from build123d import *

# Parameters (mm, degrees)
F0_R      = 9.525
F1_DEPTH  = 15.8115
F2_R      = 11.1125
F3_DEPTH  = 7.112
F4_R      = 11.1125
F5_DEPTH  = 7.112
F6_T      = 3.175
F7_R      = 3.175
F8_DEPTH  = 3.175
F10_R     = 11.1125
F11_DEPTH = 1.5875
F12_W     = 13.096875
F12_H     = 13.096875
F13_DEPTH = 15.8115
F14_R     = 4.7625
F15_R     = 8.334375


# Not quite as in the source:
# - a shell that OpenCascade refuses in one call is made with other operations: the cavity is built on its own and cut out


with BuildPart() as f1:
    # F0 (on Top) → F1 (new body)
    with BuildSketch(Plane.XY):
        with BuildLine():
            Line((-14.2875, 369.1638474552), (-14.2875, 0))
            ThreePointArc((-14.2875, 0), (-13.1999288208, -5.4675895399), (-10.1027881362, -10.1027881362))
            Line((-10.1027881362, -10.1027881362), (23.8125, -44.0180762724))
            Line((23.8125, -44.0180762724), (74.6125, -44.0180762724))
            Line((74.6125, -44.0180762724), (74.6125, 413.1819237276))
            Line((74.6125, 413.1819237276), (23.8125, 413.1819237276))
            Line((23.8125, 413.1819237276), (-10.1027881362, 379.2666355914))
            ThreePointArc((-10.1027881362, 379.2666355914), (-13.1999288208, 374.6314369951), (-14.2875, 369.1638474552))
        make_face()
        Circle(F0_R, mode=Mode.SUBTRACT)
        with Locations((0, 369.1638474552)):
            Circle(F0_R, mode=Mode.SUBTRACT)
    extrude(amount=F1_DEPTH)

    # F2 (on face) → F3 (cut)
    with BuildSketch(Plane.XY.offset(15.8115)):
        with Locations((0, 369.1638474552)):
            Circle(F2_R)
        Circle(F2_R)
    extrude(amount=-F3_DEPTH, mode=Mode.SUBTRACT)

    # F4 (on face) → F5 (cut)
    with BuildSketch(Plane(origin=(0, 0, 0), x_dir=(1, 0, 0), z_dir=(0, 0, -1))):
        Circle(F4_R)
        with Locations((0, -369.1638474552)):
            Circle(F4_R)
    extrude(amount=-F5_DEPTH, mode=Mode.SUBTRACT)

    # F6: shell of thickness 3.175, made by hand


with BuildPart() as f6_core1:
    # F6_t2: copy of F1
    add(f1.part)

    # the walls: a layer under each face that stays
    f6_faces = [f6_core1.faces().sort_by_distance(p)[0] for p in [
        (-13.1999288208, 374.6314369951, 7.90575),
        (6.8548559319, 396.2242796595, 7.90575),
        (-14.2875, 184.5819237276, 7.90575),
        (30.1625, 184.5819237276, 15.8115),
        (49.2125, 413.1819237276, 7.90575),
        (-13.1999288208, -5.4675895399, 7.90575),
        (74.6125, 184.5819237276, 7.90575),
        (6.8548559319, -27.0604322043, 7.90575),
        (49.2125, -44.0180762724, 7.90575),
        (-11.1125, 0, 3.556),
        (-11.1125, 369.1638474552, 3.556),
        (-11.1125, 0, 12.2555),
        (-11.1125, 369.1638474552, 12.2555),
        (-7.4083333333, 7.4083333333, 7.112),
        (-7.4083333333, 376.5721807885, 7.112),
        (-7.4083333333, -7.4083333333, 8.6995),
        (-7.4083333333, 361.7555141219, 8.6995),
        (-9.525, 0, 7.90575),
        (-9.525, 369.1638474552, 7.90575),
    ]]
    thicken(f6_faces, amount=-F6_T, mode=Mode.SUBTRACT)

    # F6_s3 → F6_t4 (revolve, cut)
    with BuildSketch(Plane.XZ):
        Polygon((11.08075, 7.08025), (14.2875, 7.112), (14.2875, 10.287), (11.1125, 10.287), align=None)
    revolve(axis=Axis((0, 0, 7.112), (0, 0, -1)), mode=Mode.SUBTRACT)

    # F6_s5 → F6_t6 (revolve, cut)
    with BuildSketch(Plane.XZ.offset(-369.1638474552)):
        Polygon((11.08075, 7.08025), (14.2875, 7.112), (14.2875, 10.287), (11.1125, 10.287), align=None)
    revolve(axis=Axis((0, 369.1638474552, 7.112), (0, 0, -1)), mode=Mode.SUBTRACT)

    # F6_s7 → F6_t8 (revolve, cut)
    with BuildSketch(Plane.XZ):
        Polygon((11.08075, 8.73125), (14.2875, 8.6995), (14.2875, 5.5245), (11.1125, 5.5245), align=None)
    revolve(axis=Axis((0, 0, 8.6995), (0, 0, 1)), mode=Mode.SUBTRACT)

    # F6_s9 → F6_t10 (revolve, cut)
    with BuildSketch(Plane.XZ.offset(-369.1638474552)):
        Polygon((11.08075, 8.73125), (14.2875, 8.6995), (14.2875, 5.5245), (11.1125, 5.5245), align=None)
    revolve(axis=Axis((0, 369.1638474552, 8.6995), (0, 0, 1)), mode=Mode.SUBTRACT)


with BuildPart() as f1_1:
    add(f1.part)

    # what is left inside the walls is the cavity
    f6_cavity = [f6_core1.part.solids().sort_by_distance(p)[0] for p in [
        (30.1625, 109.440257, 12.60475),
    ]]
    add(f6_cavity, mode=Mode.SUBTRACT)

    # F7
    f7_edges = [f1_1.edges().sort_by_distance(p)[0] for p in [
        (-1.507724, 383.371572, 6.31825),
        (-11.1125, 360.183591, 6.31825),
        (-11.1125, 8.980256, 6.31825),
        (-1.507724, -14.207724, 6.31825),
    ]]
    fillet(f7_edges, radius=F7_R)

    # F8 (cut, through all): a face of the model
    f8_faces = [f1_1.faces().sort_by_distance(p)[0] for p in [
        (32.2546535053, 184.5819237276, 12.6365),
    ]]
    extrude(f8_faces, amount=-F8_DEPTH, mode=Mode.SUBTRACT)

    # F10 (on offset) → F11 (join, symmetric)
    with BuildSketch(Plane.XY.offset(7.90575)):
        with BuildLine():
            Line((74.6125, -44.0180762724), (74.6125, 413.1819237276))
            Line((74.6125, 413.1819237276), (23.8125, 413.1819237276))
            Line((23.8125, 413.1819237276), (-10.1027881362, 379.2666355914))
            ThreePointArc((-10.1027881362, 379.2666355914), (-13.1999288208, 374.6314369951), (-14.2875, 369.1638474552))
            Line((-14.2875, 369.1638474552), (-14.2875, 0))
            ThreePointArc((-14.2875, 0), (-13.1999288208, -5.4675895399), (-10.1027881362, -10.1027881362))
            Line((-10.1027881362, -10.1027881362), (23.8125, -44.0180762724))
            Line((23.8125, -44.0180762724), (74.6125, -44.0180762724))
        make_face()
        Circle(F10_R, mode=Mode.SUBTRACT)
        with Locations((0, 369.1638474552)):
            Circle(F10_R, mode=Mode.SUBTRACT)
    extrude(amount=F11_DEPTH, both=True)

    # F12 (on face) → F13 (join, through all)
    with BuildSketch(Plane(origin=(0, 0, 0), x_dir=(1, 0, 0), z_dir=(0, 0, -1))):
        with Locations((68.0640625, -406.6334862276)):
            Rectangle(F12_W, F12_H)
        with Locations((68.0640625, 37.4696387724)):
            Rectangle(F12_W, F12_H)
    extrude(amount=-F13_DEPTH)

    # F14
    f14_edges = [f1_1.edges().sort_by_distance(p)[0] for p in [
        (61.515625, 400.085049, 12.652375),
        (61.515625, 400.085049, 3.159125),
        (61.515625, -30.921201, 12.652375),
        (61.515625, -30.921201, 3.159125),
    ]]
    fillet(f14_edges, radius=F14_R)

    # F15
    f15_edges = [f1_1.edges().sort_by_distance(p)[0] for p in [
        (74.6125, -44.018076, 7.90575),
        (74.6125, 413.181924, 7.90575),
    ]]
    fillet(f15_edges, radius=F15_R)


solid = f1_1.part
The model under review builds one solid part; all positions refer to its coordinate system, in mm. A direction names the side the tool comes from. Round coordinates to 2 decimals unless told otherwise and drop trailing zeros. Write each loop counter-clockwise with the first axis right and the second up, starting at its lowest first coordinate (ties: lowest second). Pieces come first, ordered by that corner, then holes. Notation, with made-up numbers: (64, -29.5) - (115, -29.5) arc R7 cw to (115, -25.5) - close; hole circle Ø3 at (42, 61.25). An arc over 180 degrees is marked (long way). One line per item, written item: value. Start each with the question number.
1. Machinability: for faces 1 (the face through (74.612, 181, 8)), 2 (the face through (13.323, 5.161, 3.203)), 3 (the face through (-5, 8.3, 8.7)), which of the approach directions +Z, -Z, +X, -X, +Y, -Y give a long, thin tool a straight path to every point of the face, cutting with its end or side? Answer none if there is none.
2. To check wall thickness, follow L1, parallel to X at y = 0, z = 1.75; L2, parallel to X at y = 147, z = 13; L3, parallel to Y at x = 0, z = 7.7 (3 decimals). State the ranges of each line that lie inside material, in increasing order. Write a range as from..to.
3. Consider section B-B on x = 40. Write out the cut boundary in (y, z).
4. Consider section A-A on y = 33.5. Write out the cut boundary in (x, z).
5. The part is to be moulded in two halves that separate along Y. For faces 4 (the face through (10.6, -3.34, 3.51)), 5 (the face through (-1.24, 378.608, 7.895)), 6 (the face through (7.09, 396.46, 8.02)), 7 (the face through (-14.288, 187, 8)), say which applies: released by +Y, released by -Y, zero draft, split by the parting line, or undercut.
6. Clearance check with flat-ended pins moving along their axes: P1, Ø1.5, axis at x = 68.5, z = 13.5, coming from the +Y side; P2, Ø10, axis at x = 56.5, y = 148.5, coming from the +Z side; P3, Ø18, axis at x = 0, y = 0, coming from the +Z side; P4, Ø2, axis at x = 5, y = 127.5, coming from the -Z side. State where each tip first meets the part, or that it passes through.
7. Consider section C-C on z = 12. State how many separate pieces and enclosed holes the cut face has, and give its area (3 significant figures).
Checks:
1. face 1: +Z, -Z, +X, +Y, -Y
1. face 2: -Z
1. face 3: +Z
2. L1: x = -14.29..-11.11, 11.11..14.29, 71.44..74.61
2. L2: x = -14.29..-11.11, 71.44..74.61
2. L3: y = -20.206..-9.525, 9.525..359.639, 378.689..389.369
3. outline: (-44.02, 0) - (-40.84, 0) - (-40.84, 6.32) - (410.01, 6.32) - (410.01, 0) - (413.18, 0) - (413.18, 15.81) - (410.01, 15.81) - (410.01, 9.49) - (-40.84, 9.49) - (-40.84, 15.81) - (-44.02, 15.81) - close
4. outline: (-14.29, 0) - (-11.11, 0) - (-11.11, 6.32) - (71.44, 6.32) - (71.44, 0) - (74.61, 0) - (74.61, 15.81) - (71.44, 15.81) - (71.44, 9.49) - (-11.11, 9.49) - (-11.11, 15.81) - (-14.29, 15.81) - close
5. face 4: undercut
5. face 5: undercut
5. face 6: released by +Y
5. face 7: zero draft
6. P1: stops at y = 413.05
6. P2: stops at z = 9.49
6. P3: passes through
6. P4: stops at z = 6.32
7. separate pieces: 1
7. enclosed holes: 3
7. area: 3,840 mm^2
